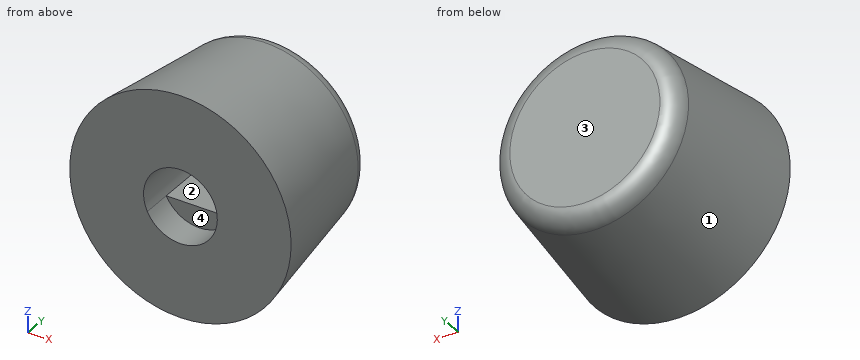
```python
from build123d import *

# Parameters (mm, degrees)
SKETCH1_R           = 9.525
BOSS_EXTRUDE1_DEPTH = 12.7
BOSS_EXTRUDE1_TAPER = 7.5
CUT_EXTRUDE1_DEPTH  = 9.525
SKETCH3_R           = 3.175
CUT_EXTRUDE2_DEPTH  = 2.54
FILLET3_R           = 1.5875


with BuildPart() as part:
    # Sketch1 → Boss-Extrude1 (new body)
    with BuildSketch(Plane(origin=(0, 0, 0), x_dir=(1, 0, 0), z_dir=(0, 1, 0))):
        Circle(SKETCH1_R)
    extrude(amount=BOSS_EXTRUDE1_DEPTH, taper=BOSS_EXTRUDE1_TAPER)

    # Sketch2 → Cut-Extrude1 (cut)
    with BuildSketch(Plane.XZ):
        with BuildLine():
            Line((-2.851142929, -1.397), (2.851142929, -1.397))
            ThreePointArc((2.851142929, -1.397), (0, 3.175), (-2.851142929, -1.397))
        make_face()
    extrude(amount=-CUT_EXTRUDE1_DEPTH, mode=Mode.SUBTRACT)

    # Sketch3 → Cut-Extrude2 (cut)
    with BuildSketch(Plane.XZ):
        with Locations(Location((0, 0, 0), (0, 0, 270))):
            Circle(SKETCH3_R)
    extrude(amount=-CUT_EXTRUDE2_DEPTH, mode=Mode.SUBTRACT)

    # Fillet3
    fillet3_edges = [part.edges().sort_by_distance(p)[0] for p in [
        (-7.853013281, 12.7, 0),
    ]]
    fillet(fillet3_edges, radius=FILLET3_R)


solid = part.part
```
Verification items for the finished model (mm, model axes). Face numbers are marked on the shaded views. Coordinates: 2 decimals unless noted, no trailing zeros. Order: outer loops, then holes, each group sorted by start corner. A loop starts at its lowest first (then second) coordinate and runs counter-clockwise, first axis right, second up. Notation, with made-up numbers: (27, -23) -> (38, -23) arc R22 ccw to (38, 5) -> close; hole circle Ø9 at (-11.5, 11). An arc over 180 degrees is marked (long way). Put each result on its own line as item: value. Start each with the question number.
1) Cross-section at B-B (y = 7). Enter the section's corners in (x, z) (3 decimals), plus the area to 3 significant figures.
2) Material ranges on L1, parallel to Z at x = -1, y = 6.5; L2, parallel to Z at x = 2.25, y = 6.25; L3, parallel to X at y = 8.75, z = 2, recorded low to high.
3) Release check for a two-part mould opening along Z. For the marked faces 1, 2, 3 and 4 record: pulls with the +Z half, pulls with the -Z half, needs draft (parallel to the pull), parting line crosses it, or undercut.
4) Cross-section at A-A (x = 0). Enter the section's corners in (y, z) (1 decimal), plus the area to 3 significant figures.
5) Go/stop test with flat-tipped pins: pin 1 (4 mm diameter, centred on y = 11, z = -6, fed in from -X); pin 2 (1.4 mm diameter, centred on x = 1, z = 1, fed in from -Y) (3 decimals); pin 3 (1 mm diameter, centred on x = -4.5, y = 5.5, fed in from -Z). Record where each tip stops, or that it passes through.
6) Cross-section at C-C (y = 8.75). Enter the section's corners in (x, z) (3 decimals).
Geometry check:
1. outline: circle Ø17.207 at (0, 0); hole (-2.851, -1.397) -> (2.851, -1.397) arc R3.175 ccw (long way) to start
1. area: 208 mm^2
2. L1: z = -8.61 to -1.4, 3.01 to 8.61
2. L2: z = -8.41 to -1.4, 2.24 to 8.41
2. L3: x = -8.13 to -2.47, 2.47 to 8.13
3. face 1: parting line crosses it
3. face 2: undercut
3. face 3: needs draft
3. face 4: undercut
4. outline: (0, -9.5) -> (11.3, -8) arc R1.6 ccw to (12.7, -6.5) -> (12.7, 6.5) arc R1.6 ccw to (11.3, 8) -> (0, 9.5) -> (0, 3.2) -> (9.5, 3.2) -> (9.5, -1.4) -> (2.5, -1.4) -> (2.5, -3.2) -> (0, -3.2) -> close
4. area: 172 mm^2
5. pin 1: stops at x = -7.06
5. pin 2: stops at y = 9.525
5. pin 3: stops at z = -7.85
6. outline: circle Ø16.746 at (0, 0); hole (-2.851, -1.397) -> (2.851, -1.397) arc R3.175 ccw (long way) to start
